Can you work these out from the model? Positions are in its coordinate system, mm. Round coordinates to 2 decimals unless told otherwise and drop trailing zeros. Loops run counter-clockwise (first coordinate to the right, second up) from the corner with the lowest first, then second, coordinate; pieces in that order, holes last. Notation, with made-up numbers: M 63,67 L 105,67 A23 cw 105,76 Z; hole C 15,38.25 d6. An arc over 180 degrees is marked long. Return JSON: item names as keys, results as strings.
```python
from build123d import *

# Parameters (mm, degrees)
F0_R     = 19.82
F1_DEPTH = 7.6
F3_DEPTH = 3.9
F5_DEPTH = 3.6


with BuildPart() as f1:
    # F0 (on Front) → F1 (new body)
    with BuildSketch(Plane.XZ):
        Circle(F0_R)
    extrude(amount=F1_DEPTH)

    # F2 (on face) → F3 (cut)
    with BuildSketch(Plane.XZ.offset(7.6)):
        Polygon((-3.775, 3.9), (-21.085563, 3.9), (-21.085563, -3.9), (-3.775, -3.9), (-3.775, -6.875), (3.775, -6.875), (3.775, -3.9), (21.085563, -3.9), (21.085563, 3.9), (3.775, 3.9), (3.775, 6.875), (-3.775, 6.875), align=None)
    extrude(amount=-F3_DEPTH, mode=Mode.SUBTRACT)

    # F4 (on Front) → F5 (join)
    with BuildSketch(Plane.XZ):
        Polygon((-4.025, 24.657003), (-4.025, 19.407003), (-1.575, 19.407003), (-1.575, 22.257003), (1.525, 22.257003), (1.525, 20.657003), (4.025, 20.657003), (4.025, 24.657003), align=None)
    extrude(amount=F5_DEPTH)


solid = f1.part
```
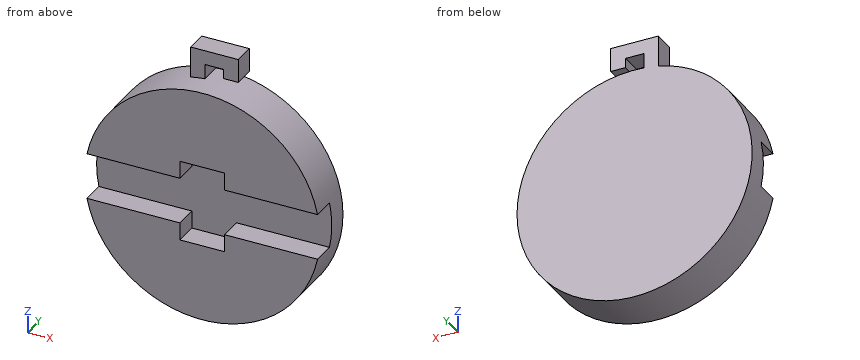
Q1. If I drill on line 1 along Z through (x, y) = (-9, -6.25); line 2 along Z through (x, y) = (5.5, -6.25); line 3 along Y through (x, z) = (16, -1.5), over which ranges is the centre line in solid material (lowest first)?
Results:
{"line 1": "z = -17.66 to -3.9, 3.9 to 17.66", "line 2": "z = -19.04 to -3.9, 3.9 to 19.04", "line 3": "y = -3.7 to 0"}
Q2. Suppose I cut it at A-A, the plane x = 0. Please give me the cut outline in (y, z) (3 decimals).
Results:
{"outline": "M -7.6,-19.82 L 0,-19.82 L 0,19.82 L -7.6,19.82 L -7.6,6.875 L -3.7,6.875 L -3.7,-6.875 L -7.6,-6.875 Z; M -3.6,22.257 L 0,22.257 L 0,24.657 L -3.6,24.657 Z"}
Q3. Suppose I cut it at C-C, the plane z = -5.5. Please give me the cut outline in (x, y) (3 decimals).
Results:
{"outline": "M -19.042,-7.6 L -3.775,-7.6 L -3.775,-3.7 L 3.775,-3.7 L 3.775,-7.6 L 19.042,-7.6 L 19.042,0 L -19.042,0 Z"}
Q4. Suppose I cut it at B-B, the plane y = -5.75. Please give me the cut outline in (x, z) (1 decimal).
Results:
{"outline": "M -19.4,-3.9 A19.8 ccw 19.4,-3.9 L 3.8,-3.9 L 3.8,-6.9 L -3.8,-6.9 L -3.8,-3.9 Z; M -19.4,3.9 L -3.8,3.9 L -3.8,6.9 L 3.8,6.9 L 3.8,3.9 L 19.4,3.9 A19.8 ccw Z"}
Q5. I'm going to push flat-ended pins straight in: pin 1 Ø1.8 at (y, z) = (-2.5, 23) entering from +X (3 decimals); pin 2 Ø1.5 at (y, z) = (-6, 5) entering from +X; pin 3 Ø1.3 at (y, z) = (-1, 21.5) entering from -X (3 decimals). Where does each tip first touch, or does it pass through?
Results:
{"pin 1": "stops at x = 4.025", "pin 2": "stops at x = 19.36", "pin 3": "stops at x = -4.025"}
Q6. Suppose I cut it at D-D, the plane x = -7. Please give me the cut outline in (y, z), plus the area to 3 significant figures.
Results:
{"outline": "M -7.6,-18.54 L 0,-18.54 L 0,18.54 L -7.6,18.54 L -7.6,3.9 L -3.7,3.9 L -3.7,-3.9 L -7.6,-3.9 Z", "area": "251 mm2"}
